For this review, take the finished solid that the model builds, in its own axes (mm). A direction names the side the tool comes from. Give positions to 0.01 mm unless a question says otherwise; leave off trailing zeros. Loops run counter-clockwise (first coordinate to the right, second up) from the corner with the lowest first, then second, coordinate; pieces in that order, holes last.
```python
from build123d import *

# Parameters (mm, degrees)
SKETCH1_W           = 30
SKETCH1_H           = 20
BOSS_EXTRUDE1_DEPTH = 1.25
SKETCH2_W           = 5
SKETCH2_H           = 20
BOSS_EXTRUDE2_DEPTH = 71
BOSS_EXTRUDE3_DEPTH = 20
CUT_EXTRUDE2_REACH  = 3.25
SKETCH4_R           = 1.5
FILLET1_R           = 2


with BuildPart() as part:
    # Sketch1 → Boss-Extrude1 (new body)
    with BuildSketch(Plane(origin=(0, 0, 0), x_dir=(1, 0, 0), z_dir=(0, 1, 0))):
        Rectangle(SKETCH1_W, SKETCH1_H)
    extrude(amount=BOSS_EXTRUDE1_DEPTH)

    # Sketch2 → Boss-Extrude2 (add)
    with BuildSketch(Plane(origin=(0, 1.25, 0), x_dir=(1, 0, 0), z_dir=(0, 1, 0))):
        with Locations((3.5, 0)):
            Rectangle(SKETCH2_W, SKETCH2_H)
    extrude(amount=BOSS_EXTRUDE2_DEPTH)

    # Sketch3 → Boss-Extrude3 (add)
    with BuildSketch(Plane.XY.offset(10)):
        Polygon((1, 36.25), (-11.805511119, 1.25), (-15, 1.25), (1, 44.981171275), align=None)
    extrude(amount=-BOSS_EXTRUDE3_DEPTH)

    # Sketch4 → Cut-Extrude2 (cut, up to next)
    with BuildSketch(Plane(origin=(0, 1.25, 0), x_dir=(1, 0, 0), z_dir=(0, 1, 0)), mode=Mode.PRIVATE) as cut_extrude2_sk1:
        with Locations((9.5, 0)):
            Circle(SKETCH4_R)
    cut_extrude2_tool1 = extrude(cut_extrude2_sk1.sketch, amount=-CUT_EXTRUDE2_REACH, mode=Mode.PRIVATE) & part.part
    add(cut_extrude2_tool1.solids().sort_by_distance((9.5, 1.25, 0))[0], mode=Mode.SUBTRACT)

    # Fillet1
    fillet1_edges = [part.edges().sort_by_distance(p)[0] for p in [
        (3.5, 72.25, -10),
        (3.5, 72.25, 10),
        (1, 44.981171275, 0),
    ]]
    fillet(fillet1_edges, radius=FILLET1_R)


solid = part.part
```
Item 1: Tool access review of faces 4 (the flat face through (6, 36, 0)), 5 (the flat face through (1, 59, 0)), 6 (the flat face through (1, 19, 0)): name each direction out of +Z, -Z, +X, -X, +Y, -Y from which nothing blocks a thin tool from reaching the whole face with its end or side.
Answer:
face 4: +Z, -Z, +X, +Y
face 5: +Z, -Z, -X, +Y
face 6: +Z, -Z
Item 2: For L1, parallel to Z at x = 9.5, y = 1; L2, parallel to Y at x = 7.75, z = 7.5; L3, parallel to X at y = 0.4, z = 0, list the stretches that pass through material, from the lowest coordinate up.
Answer:
L1: z = -10 to -1.5, 1.5 to 10
L2: y = 0 to 1.25
L3: x = -15 to 8, 11 to 15
Item 3: The part is to be moulded in two halves that separate along Y. For faces 1 (the flat face through (-5.313, 18.995, 0.14)), 2 (the flat face through (1.2, 30.1, -10)), 3 (the flat face through (11.4, 1.25, -0.1)), say which applies: released by +Y, released by -Y, zero draft, split by the parting line, or undercut.
Answer:
face 1: undercut
face 2: zero draft
face 3: released by +Y
Item 4: Take a section at C-C on y = 10. Give the boundary of the cut face in (x, z), and give its area (3 significant figures).
Answer:
outline: (-11.8, -10) - (-8.6, -10) - (-8.6, 10) - (-11.8, 10) - close; (1, -10) - (6, -10) - (6, 10) - (1, 10) - close
area: 164 mm2
Item 5: Clearance check with flat-ended pins moving along their axes: pin 1 Ø3.5 at (x, z) = (9.5, 0) entering from +Y; pin 2 Ø8 at (y, z) = (15.5, 3) entering from +X; pin 3 Ø10 at (y, z) = (15, -1.5) entering from -X. State where each tip first meets the part, or that it passes through.
Answer:
pin 1: stops at y = 1.25
pin 2: stops at x = 6
pin 3: stops at x = -11.8
Item 6: Take a section at A-A on z = 0. Give the boundary of the cut face in (x, y).
Answer:
outline: (-15, 0) - (8, 0) - (8, 1.25) - (6, 1.25) - (6, 72.25) - (1, 72.25) - (1, 45.34) arc R2 cw to (0.88, 44.65) - (-15, 1.25) - close; (11, 0) - (15, 0) - (15, 1.25) - (11, 1.25) - close; hole (-11.81, 1.25) - (1, 1.25) - (1, 36.25) - close
Item 7: Take a section at B-B on x = 9.5. Give the boundary of the cut face in (y, z).
Answer:
outline: (0, -10) - (1.25, -10) - (1.25, -1.5) - (0, -1.5) - close; (0, 1.5) - (1.25, 1.5) - (1.25, 10) - (0, 10) - close
Item 8: Take a section at D-D on x = 13. Give the boundary of the cut face in (y, z).
Answer:
outline: (0, -10) - (1.25, -10) - (1.25, 10) - (0, 10) - close
